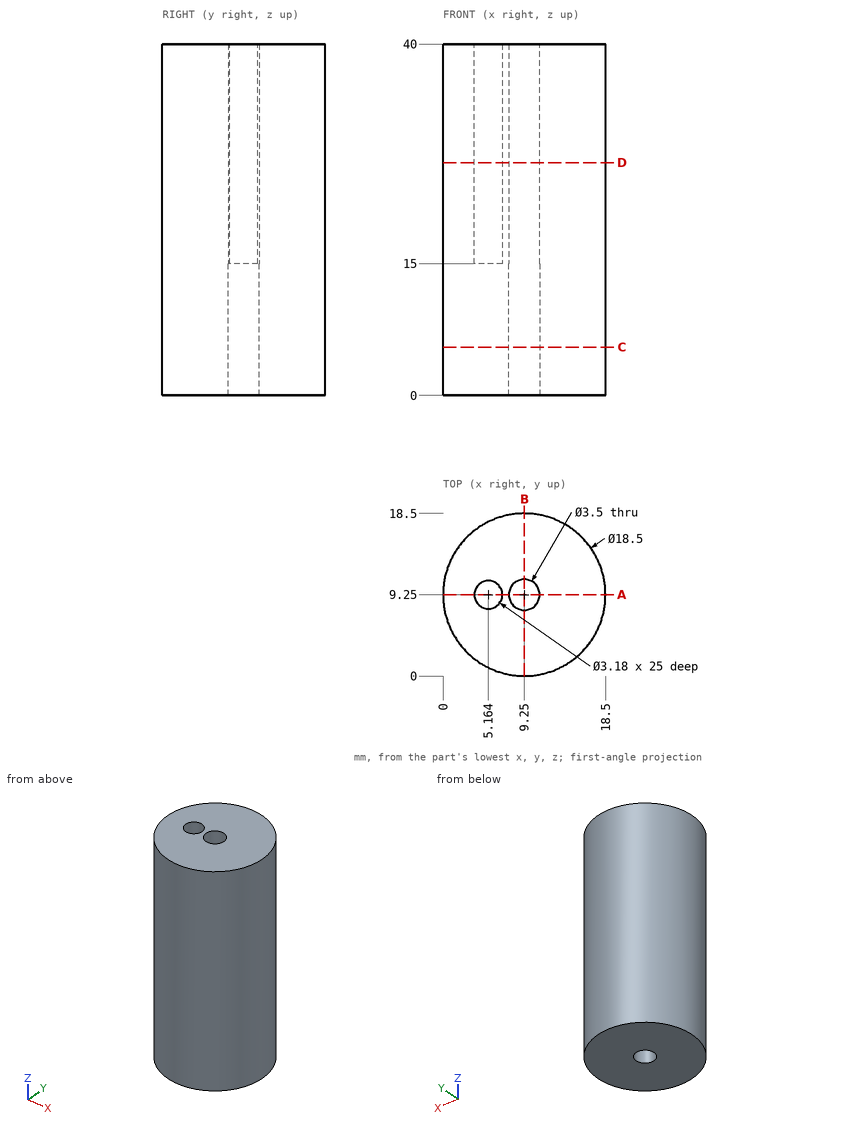
Geometry: see drawing. Coordinates: mm, zero at the bounding-box minimum. Coordinates: 2 decimals unless noted, no trailing zeros. Write each loop counter-clockwise with the first axis right and the second up, starting at its lowest first coordinate (ties: lowest second). Pieces come first, ordered by that corner, then holes.
1) Pin query (flat end, axial travel): pin 1 Ø1 at (x, z) = (9, 26.5) entering from +Y; pin 2 Ø1 at (x, z) = (11.5, 29.5) entering from -Y; pin 3 Ø6 at (x, z) = (3.5, 30) entering from +Y; pin 4 Ø4 at (y, z) = (3, 22) entering from +X (1 decimal). Return the tip coordinate at first contact, or that it passes through.
2) Section B-B on x = 9.25. Output: boundary loops of the cut face in (y, z).
3) Section D-D on z = 26.5. State how many separate pieces and enclosed holes the cut face has, and give its area (3 significant figures).
4) Section A-A on y = 9.25. Output: boundary loops of the cut face in (x, z) (1 decimal).
5) Section C-C on z = 5.5. Output: boundary loops of the cut face in (x, y).
6) Material intervals for line 1 along Y through (x, z) = (9.25, 6.25); line 2 along X through (y, z) = (10.25, 30) (1 decimal); line 3 along Y through (x, z) = (10.25, 13.5) (1 decimal), sorted ascending.
Check result:
1. pin 1: stops at y = 18.5
1. pin 2: stops at y = 0.17
1. pin 3: stops at y = 18.08
1. pin 4: stops at x = 17.5
2. outline: (0, 0) - (7.5, 0) - (7.5, 40) - (0, 40) - close; (11, 0) - (18.5, 0) - (18.5, 40) - (11, 40) - close
3. separate pieces: 1
3. enclosed holes: 2
3. area: 251 mm2
4. outline: (0, 0) - (7.5, 0) - (7.5, 40) - (6.8, 40) - (6.8, 15) - (3.6, 15) - (3.6, 40) - (0, 40) - close; (11, 0) - (18.5, 0) - (18.5, 40) - (11, 40) - close
5. outline: circle Ø18.5 at (9.25, 9.25); hole circle Ø3.5 at (9.25, 9.25)
6. line 1: y = 0 to 7.5, 11 to 18.5
6. line 2: x = 0.1 to 3.9, 6.4 to 7.8, 10.7 to 18.4
6. line 3: y = 0.1 to 7.8, 10.7 to 18.4
